The model under review builds one solid part; all positions refer to its coordinate system, in mm. A direction names the side the tool comes from. Round coordinates to 2 decimals unless told otherwise and drop trailing zeros. Order: outer loops, then holes, each group sorted by start corner. A loop starts at its lowest first (then second) coordinate and runs counter-clockwise, first axis right, second up.
1) Machinability: for faces 4 (the face through (-2, 51, -1)), 5 (the face through (-13, 49, -3)), which of the approach directions +Z, -Z, +X, -X, +Y, -Y give a long, thin tool a straight path to every point of the face, cutting with its end or side? Answer none if there is none.
2) Mouldability with a two-part tool opening along Z and no side actions: class faces 1 (the face through (-12, 49, 0)), 2 (the face through (-1.48, 5.98, -14.16)), 3 (the face through (-20, 49, -1)) as pulls with the +Z half, pulls with the -Z half, needs draft (parallel to the pull), parting line crosses it, or undercut.
3) Consider section A-A (y = 7.5). Give the boundary of the cut face in (x, z), then the cut area to 3 significant figures.
4) Clearance check with a flat-ended pin moving along its axis: P1, Ø5, axis at y = 24, z = -15.5, coming from the -X side. State where the tip first meets the part, or that it passes through.
5) Consider section C-C (x = -12.5). Give the boundary of the cut face in (y, z).
6) Consider section B-B (z = -12.5). Give the boundary of the cut face in (x, y), then the cut area to 3 significant figures.
7) To check wall thickness, follow L1, parallel to Y at x = -0.7, z = -12.5; L2, parallel to X at y = 59, z = -13.75; L3, parallel to Z at x = -1.15, y = 92.5. State the ranges of each line that lie inside material, in increasing order.
8) Consider section D-D (y = 89). Give the boundary of the cut face in (x, z).
Autodesk Inventor part; units mm, degrees
ref_plane "YZ Plane" through (0, 0, 0) normal (1, 0, 0) x (0, 1, 0)
ref_plane "XZ Plane" through (0, 0, 0) normal (0, 1, 0) x (-1, 0, 0)
ref_plane "XY Plane" through (0, 0, 0) normal (0, 0, 1) x (1, 0, 0)
sketch "Sketch1" plane through (0, 0, 0) normal (0, 1, 0) x (-1, 0, 0)
  line L0 (0, 0) -> (20, 0)
  line L1 (20, 0) -> (20, -3)
  line L2 (20, -3) -> (0, -3)
  line L3 (0, -3) -> (0, 0)
  line L4 (0, 0) -> (3, 0)
  line L5 (3, 0) -> (3, -20)
  line L6 (3, -20) -> (0, -20)
  line L7 (0, -20) -> (0, 0)
  dimension "d0" = 3
  dimension "d1" = 3
  dimension "d2" = 20
  dimension "d3" = 20
extrude "Extrusion1" add sketch "Sketch1" along normal blind 100
fillet "Fillet1" radius 2 1 edges at (-3, 50, -3)
fillet "Fillet2" radius 5 1 edges at (0, 50, 0)
sketch "Sketch2" plane through (-3, 0, -20) normal (-1, 0, 0) x (0, 0, 1)
  line L0 (0, 100) -> (15, 100)
  line L1 (0, 0) -> (15, 0)
  line L2 (0, 0) -> (0, 100)
  point P0 (20, 0)
  point P1 (7.5, 92.5)
  point P2 (7.5, 7.5)
  dimension "d8" = 7.5
  dimension "d9" = 7.5
  dimension "d10" = 85
  dimension "d11" = 7.5
hole "Hole1" at (-3, 92.5, -12.5) at (-3, 7.5, -12.5) direction (1, 0, 0) diameter 4.5 end through all
sketch "Sketch3" plane through (-20, 0, -3) normal (0, 0, -1) x (-1, 0, 0)
  line L0 (-15, 100) -> (0, 100)
  line L1 (-15, 0) -> (0, 0)
  line L2 (0, 0) -> (0, 100)
  point P0 (-20, 0)
  point P1 (-7.5, 92.5)
  point P2 (-7.5, 7.5)
  dimension "d19" = 7.5
  dimension "d20" = 7.5
  dimension "d21" = 7.5
hole "Hole2" at (-12.5, 92.5, -3) at (-12.5, 7.5, -3) direction (0, 0, 1) diameter 4.5 end through all
equation "\"d1\" = d0"
equation "\"d3\" = d2"
properties part number "Pancake_Angle Bracket 2" material "Aluminum 6061"
Answer below:
1. face 4: +Z, +X, +Y, -Y
1. face 5: -Z, -X, +Y, -Y
2. face 1: pulls with the +Z half
2. face 2: undercut
2. face 3: needs draft
3. outline: (-20, -3) - (-14.75, -3) - (-14.75, 0) - (-20, 0) - close; (-10.25, -3) - (-5, -3) arc R2 cw to (-3, -5) - (-3, -10.25) - (0, -10.25) - (0, -5) arc R5 ccw to (-5, 0) - (-10.25, 0) - close; (-3, -20) - (0, -20) - (0, -14.75) - (-3, -14.75) - close
3. area: 79.5 mm2
4. P1: stops at x = -3
5. outline: (0, -3) - (5.25, -3) - (5.25, 0) - (0, 0) - close; (9.75, -3) - (90.25, -3) - (90.25, 0) - (9.75, 0) - close; (94.75, -3) - (100, -3) - (100, 0) - (94.75, 0) - close
6. outline: (-3, 0) - (0, 0) - (0, 5.25) - (-3, 5.25) - close; (-3, 9.75) - (0, 9.75) - (0, 90.25) - (-3, 90.25) - close; (-3, 94.75) - (0, 94.75) - (0, 100) - (-3, 100) - close
6. area: 273 mm2
7. L1: y = 0 to 5.25, 9.75 to 90.25, 94.75 to 100
7. L2: x = -3 to 0
7. L3: z = -20 to -14.75, -10.25 to -1.81
8. outline: (-20, -3) - (-5, -3) arc R2 cw to (-3, -5) - (-3, -20) - (0, -20) - (0, -5) arc R5 ccw to (-5, 0) - (-20, 0) - close
